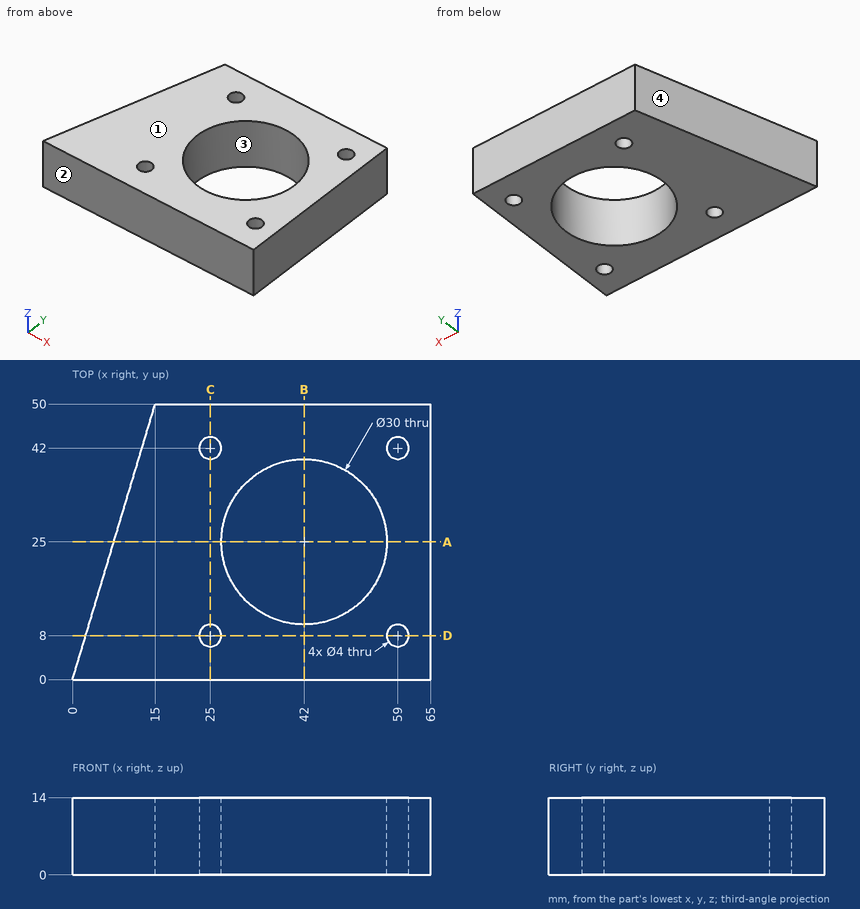
Verification items for this drawing (mm, ordinates from the low corner). Coordinates: 2 decimals unless noted, no trailing zeros. Write each loop counter-clockwise with the first axis right and the second up, starting at its lowest first coordinate (ties: lowest second). Pieces come first, ordered by that corner, then holes. Notation, with made-up numbers: M 26.5,87 L 80.5,87 A26 cw 80.5,118 Z; hole C 83,56 d8. An arc over 180 degrees is marked long. One line per item, written item: value. Start each with the question number.
(1) Scan lines: line 1 along Y through (x, z) = (42, 6.5); line 2 along X through (y, z) = (42.5, 12.75); line 3 along Y through (x, z) = (39.5, 13.25). Record each from-to range of solid material in increasing order. Write a range as [from, to].
(2) Sectioned sample at D-D, the plane y = 8. Enter the section's corners in (x, z).
(3) Release check for a two-part mould opening along Y. For the marked faces 1, 2, 3 and 4 record: released by +Y, released by -Y, zero draft, split by the parting line, or undercut.
(4) Sectioned sample at B-B, the plane x = 42. Enter the section's corners in (y, z).
(5) Sectioned sample at C-C, the plane x = 25. Enter the section's corners in (y, z), and give its area (3 significant figures).
(6) Depth check by flat-ended pin: pin 1 (1 mm diameter, centred on y = 5.5, z = 8.5, fed in from -X). Enter the tip coordinate at first touch or a pass-through.
(7) Sectioned sample at A-A, the plane y = 25. Enter the section's corners in (x, z).
Filled sheet:
1. line 1: [0, 10], [40, 50]
1. line 2: [12.75, 23.06], [26.94, 57.06], [60.94, 65]
1. line 3: [0, 10.21], [39.79, 50]
2. outline: M 2.4,0 L 23,0 L 23,14 L 2.4,14 Z; M 27,0 L 57,0 L 57,14 L 27,14 Z; M 61,0 L 65,0 L 65,14 L 61,14 Z
3. face 1: zero draft
3. face 2: released by -Y
3. face 3: undercut
3. face 4: released by +Y
4. outline: M 0,0 L 10,0 L 10,14 L 0,14 Z; M 40,0 L 50,0 L 50,14 L 40,14 Z
5. outline: M 0,0 L 6,0 L 6,14 L 0,14 Z; M 10,0 L 40,0 L 40,14 L 10,14 Z; M 44,0 L 50,0 L 50,14 L 44,14 Z
5. area: 588 mm²
6. pin 1: x = 1.5
7. outline: M 7.5,0 L 27,0 L 27,14 L 7.5,14 Z; M 57,0 L 65,0 L 65,14 L 57,14 Z
